Study the drawing (mm; zero at the part's minimum x, y, z) and answer. Coordinates: 2 decimals unless noted, no trailing zeros. Order: outer loops, then holes, each group sorted by start corner. A loop starts at its lowest first (then second) coordinate and runs counter-clockwise, first axis right, second up. Notation, with made-up numbers: (60, -38.5) -> (109, -38.5) arc R6 cw to (109, -27.5) -> close; hole circle Ø11 at (42, 75). An arc over 180 degrees is marked (long way). Write each question's results on one line, items separated by ' | '. Start each with the question number.
(1) Straight lines are drawn through the part: L1, parallel to Y at x = 88.9, z = 1.2; L2, parallel to X at y = 30.5, z = 2.75; L3, parallel to X at y = 58, z = 1.7. For each, find the intervals that lie inside material, in ascending order.
(2) The part is cut by section B-B, the plane y = 16.51. Give the vertices of the cut face in (x, z) (3 decimals).
(3) The part is cut by section C-C, the plane x = 54.61. Give the vertices of the cut face in (y, z) (3 decimals), then the cut area to 3 significant figures.
(4) The part is cut by section D-D, the plane y = 52.5. Give the vertices of the cut face in (x, z) (3 decimals), then the cut area to 3 significant figures.
(5) The part is cut by section A-A, the plane z = 0.8. Give the vertices of the cut face in (x, y), then the cut area to 3 significant figures.
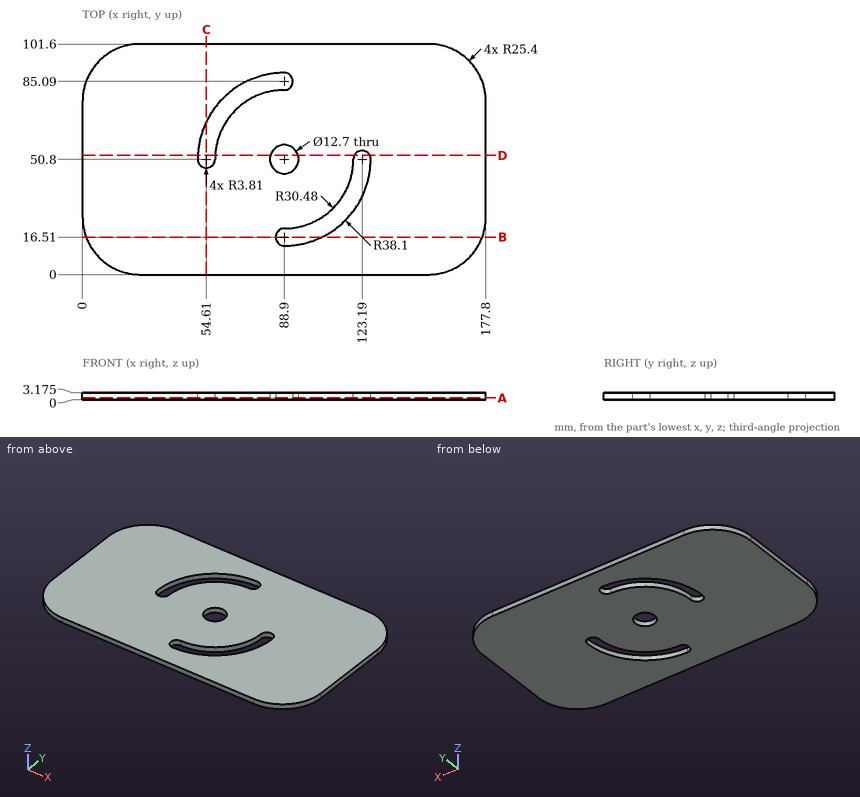
Established:
1) L1: y = 0 to 12.7, 20.32 to 44.45, 57.15 to 81.28, 88.9 to 101.6 | L2: x = 0 to 111.64, 121.14 to 177.8 | L3: x = 0 to 51.49, 59.28 to 177.8
2) outline: (1.607, 0) -> (85.09, 0) -> (85.09, 3.175) -> (1.607, 3.175) -> close; (105.507, 0) -> (176.193, 0) -> (176.193, 3.175) -> (105.507, 3.175) -> close
3) outline: (0, 0) -> (46.99, 0) -> (46.99, 3.175) -> (0, 3.175) -> close; (67.407, 0) -> (101.6, 0) -> (101.6, 3.175) -> (67.407, 3.175) -> close | area: 258 mm^2
4) outline: (0, 0) -> (50.838, 0) -> (50.838, 3.175) -> (0, 3.175) -> close; (58.467, 0) -> (82.782, 0) -> (82.782, 3.175) -> (58.467, 3.175) -> close; (95.018, 0) -> (119.78, 0) -> (119.78, 3.175) -> (95.018, 3.175) -> close; (126.6, 0) -> (177.8, 0) -> (177.8, 3.175) -> (126.6, 3.175) -> close | area: 480 mm^2
5) outline: (0, 25.4) arc R25.4 ccw to (25.4, 0) -> (152.4, 0) arc R25.4 ccw to (177.8, 25.4) -> (177.8, 76.2) arc R25.4 ccw to (152.4, 101.6) -> (25.4, 101.6) arc R25.4 ccw to (0, 76.2) -> close; hole (50.8, 50.8) arc R3.81 ccw to (58.42, 50.8) arc R30.48 cw to (88.9, 81.28) arc R3.81 ccw to (88.9, 88.9) arc R38.1 ccw to start; hole circle Ø12.7 at (88.9, 50.8); hole (88.9, 12.7) arc R38.1 ccw to (127, 50.8) arc R3.81 ccw to (119.38, 50.8) arc R30.48 cw to (88.9, 20.32) arc R3.81 ccw to start | area: 16,500 mm^2
